Drawing for the job (mm, zero at the part's lowest x, y, z). A direction names the side the tool comes from. Round coordinates to 2 decimals unless told otherwise and drop trailing zeros. Order: outer loops, then holes, each group sorted by start corner. A loop starts at its lowest first (then second) coordinate and runs counter-clockwise, first axis right, second up. Notation, with made-up numbers: (75.25, 6.5) -> (91.25, 6.5) arc R34 cw to (91.25, 36.5) -> close; hole circle Ø6 at (42, -34). An arc over 180 degrees is marked (long way). Use CSV: the item, a comma, the result in double quotes.
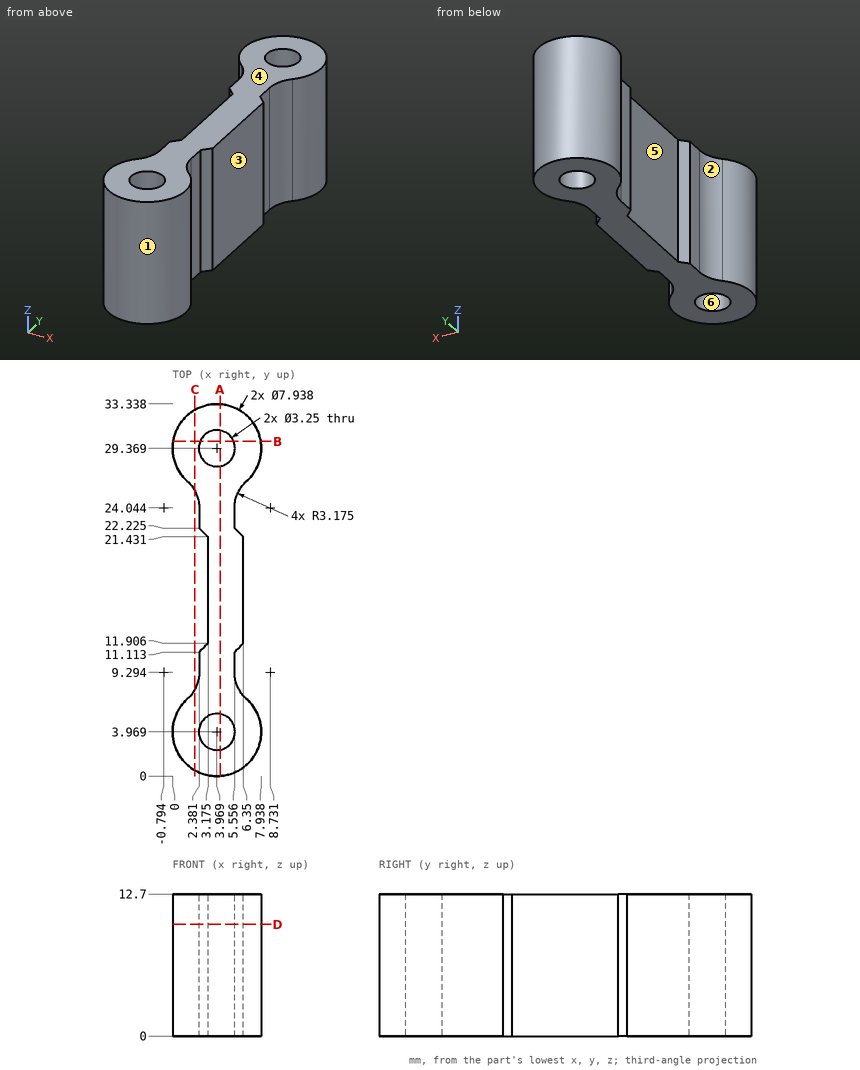
Q1. Which spindle directions (+Z, -Z, +X, -X, +Y, -Y) get a long thin tool onto all of the face, cutting with end or side? Do the marked faces 1, 2 and 3. Say none if no direction does.
From the geometry:
face 1,"+Z, -Z"
face 2,"+Z, -Z, -X"
face 3,"+Z, -Z, +X"
Q2. Cut at B-B (y = 30). Give the cut face in (x, z).
From the geometry:
outline,"(0.05, 0) -> (2.47, 0) -> (2.47, 12.7) -> (0.05, 12.7) -> close; (5.47, 0) -> (7.89, 0) -> (7.89, 12.7) -> (5.47, 12.7) -> close"
Q3. Mould opens along X. For the marked faces 4, 5 and 6 say: +X half, -X half, draft (parallel to the pull), parting line (faces both ways), or undercut.
From the geometry:
face 4,"draft"
face 5,"-X half"
face 6,"undercut"
Q4. Pin check, flat tips, straight feed: pin 1 (5 mm diameter, centred on y = 15, z = 7.5, fed in from +X); pin 2 (1.5 mm diameter, centred on y = 10.5, z = 6.5, fed in from +X) (1 decimal); pin 3 (3.5 mm diameter, centred on x = 3.97, y = 3.97, fed in from +Z); pin 4 (2 mm diameter, centred on y = 10.5, z = 7, fed in from -X). Stop position of each tip, or through.
From the geometry:
pin 1,"stops at x = 6.35"
pin 2,"stops at x = 5.7"
pin 3,"stops at z = 12.7"
pin 4,"stops at x = 2.38"
Q5. Cut at D-D (z = 10). State how many separate pieces and enclosed holes the cut face has, plus the area to 3 significant figures.
From the geometry:
separate pieces,"1"
enclosed holes,"2"
area,"140 mm²"
Q6. Cut at C-C (x = 2). Give the cut face in (y, z) (1 decimal).
From the geometry:
outline,"(0.5, 0) -> (7.8, 0) -> (7.8, 12.7) -> (0.5, 12.7) -> close; (25.6, 0) -> (32.8, 0) -> (32.8, 12.7) -> (25.6, 12.7) -> close"
Q7. Probe line 1 along Y through (x, z) = (3.25, 3.5) (1 decimal); line 2 along Y through (x, z) = (6.25, 6.25) (1 decimal); line 3 along Y through (x, z) = (2.5, 1.25) (1 decimal). List the from-to ranges inside material, lowest first.
From the geometry:
line 1,"y = 0.1 to 2.5, 5.4 to 27.9, 30.8 to 33.3"
line 2,"y = 0.7 to 7.3, 11.8 to 21.5, 26 to 32.6"
line 3,"y = 0.3 to 3.3, 4.7 to 11.2, 22.1 to 28.7, 30.1 to 33.1"
Q8. Cut at A-A (x = 4.25). Give the cut face in (y, z), plus the area to 3 significant figures.
From the geometry:
outline,"(0.01, 0) -> (2.37, 0) -> (2.37, 12.7) -> (0.01, 12.7) -> close; (5.57, 0) -> (27.77, 0) -> (27.77, 12.7) -> (5.57, 12.7) -> close; (30.97, 0) -> (33.33, 0) -> (33.33, 12.7) -> (30.97, 12.7) -> close"
area,"342 mm²"
